```python
from build123d import *

# Parameters (mm, degrees)
SKETCH1_W           = 64.08
SKETCH1_H           = 37.749
BOSS_EXTRUDE1_DEPTH = 20.32
SKETCH1_6_W         = 59
SKETCH1_6_H         = 32.669
CUT_EXTRUDE1_DEPTH  = 17.78
SKETCH4_R           = 1.75
BOSS_EXTRUDE2_DEPTH = 8.89
SKETCH6_W           = 8
SKETCH6_H           = 3
CUT_EXTRUDE2_DEPTH  = 8.89


with BuildPart() as part:
    # Sketch1 → Boss-Extrude1 (new body)
    with BuildSketch(Plane(origin=(0, 0, 0), x_dir=(1, 0, 0), z_dir=(0, 1, 0))):
        Rectangle(SKETCH1_W, SKETCH1_H)
    extrude(amount=-BOSS_EXTRUDE1_DEPTH)

    # Sketch1_6 → Cut-Extrude1 (cut)
    with BuildSketch(Plane(origin=(0, 0, 0), x_dir=(1, 0, 0), z_dir=(0, 1, 0))):
        Rectangle(SKETCH1_6_W, SKETCH1_6_H)
    extrude(amount=-CUT_EXTRUDE1_DEPTH, mode=Mode.SUBTRACT)

    # Sketch4 → Boss-Extrude2 (add)
    # profile 1 of 4: a face of its own
    with BuildSketch(Plane(origin=(0, -17.78, 0), x_dir=(1, 0, 0), z_dir=(0, 1, 0))):
        with BuildLine():
            Line((-29.5, 16.3345), (-24.3228, 16.3345))
            ThreePointArc((-24.3228, 16.3345), (-24.192690413, 11.027190413), (-29.5, 10.897080827))
            Line((-29.5, 10.897080827), (-29.5, 16.3345))
        make_face()
        with Locations(Location((-26.9114, 13.615790413, 0), (0, 0, 270))):
            Circle(SKETCH4_R, mode=Mode.SUBTRACT)
    # profile 2 of 4: a face of its own
    with BuildSketch(Plane(origin=(0, -17.78, 0), x_dir=(1, 0, 0), z_dir=(0, 1, 0))):
        with BuildLine():
            Line((29.5, 10.897080827), (29.5, 16.3345))
            Line((29.5, 16.3345), (24.3228, 16.3345))
            ThreePointArc((24.3228, 16.3345), (24.192690413, 11.027190413), (29.5, 10.897080827))
        make_face()
        with Locations(Location((26.9114, 13.615790413, 0), (0, 0, 270))):
            Circle(SKETCH4_R, mode=Mode.SUBTRACT)
    # profile 3 of 4: a face of its own
    with BuildSketch(Plane(origin=(0, -17.78, 0), x_dir=(1, 0, 0), z_dir=(0, 1, 0))):
        with BuildLine():
            Line((29.5, -10.897080827), (29.5, -16.3345))
            Line((29.5, -16.3345), (24.3228, -16.3345))
            ThreePointArc((24.3228, -16.3345), (24.192690413, -11.027190413), (29.5, -10.897080827))
        make_face()
        with Locations(Location((26.9114, -13.615790413, 0), (0, 0, 270))):
            Circle(SKETCH4_R, mode=Mode.SUBTRACT)
    # profile 4 of 4: a face of its own
    with BuildSketch(Plane(origin=(0, -17.78, 0), x_dir=(1, 0, 0), z_dir=(0, 1, 0))):
        with BuildLine():
            Line((-29.5, -10.897080827), (-29.5, -16.3345))
            Line((-29.5, -16.3345), (-24.3228, -16.3345))
            ThreePointArc((-24.3228, -16.3345), (-24.192690413, -11.027190413), (-29.5, -10.897080827))
        make_face()
        with Locations(Location((-26.9114, -13.615790413, 0), (0, 0, 270))):
            Circle(SKETCH4_R, mode=Mode.SUBTRACT)
    extrude(amount=BOSS_EXTRUDE2_DEPTH)

    # Sketch6 → Cut-Extrude2 (cut)
    with BuildSketch(Plane(origin=(32.04, 0, 0), x_dir=(0, 0, -1), z_dir=(1, 0, 0))):
        with Locations((-0.19, -7.82)):
            Rectangle(SKETCH6_W, SKETCH6_H)
    extrude(amount=-CUT_EXTRUDE2_DEPTH, mode=Mode.SUBTRACT)


solid = part.part
```
Geometry: final body of the model. Coordinates: model frame, mm. A direction names the side the tool comes from. Coordinates: 2 decimals unless noted, no trailing zeros. Order: outer loops, then holes, each group sorted by start corner. A loop starts at its lowest first (then second) coordinate and runs counter-clockwise, first axis right, second up. Notation, with made-up numbers: M 21,-15 L 46,-15 A12 ccw 46,-9 Z; hole C -1.5,83 d1. An arc over 180 degrees is marked long. Answer as CSV lines item,"result".
Q1. Section B-B on y = -4.75. Return the cut outline in (x, z).
Answers:
outline,"M -32.04,-18.87 L 32.04,-18.87 L 32.04,18.87 L -32.04,18.87 Z; hole M -29.5,-16.33 L 29.5,-16.33 L 29.5,16.33 L -29.5,16.33 Z"
Q2. Section D-D on y = -7.5. Return the cut outline in (x, z).
Answers:
outline,"M -32.04,-18.87 L 32.04,-18.87 L 32.04,-3.81 L 29.5,-3.81 L 29.5,-16.33 L -29.5,-16.33 L -29.5,16.33 L 29.5,16.33 L 29.5,4.19 L 32.04,4.19 L 32.04,18.87 L -32.04,18.87 Z"
Q3. Draft query along Z for faces 1 (the cylindrical face through (-24.136, -13.397, 11.088)), 2 (the flat face through (-3, 0, 17)), 3 (the flat face through (0, -10, -18.874)). Return one class per face: pulls with the +Z half, pulls with the -Z half, needs draft (parallel to the pull), parting line crosses it, or undercut.
Answers:
face 1,"undercut"
face 2,"needs draft"
face 3,"pulls with the -Z half"
Q4. First-contact query: P1, Ø1, axis at x = 27, z = 13.5, coming from the +Y side; P2, Ø4, axis at x = -26.91, z = 13.62, coming from the +Y side. Flat tips, straight axial feed; report the tip coordinate or a pass-through.
Answers:
P1,"stops at y = -17.78"
P2,"stops at y = -8.89"
Q5. Section A-A on z = -2. Return the cut outline in (x, y), and give its area (3 significant figures).
Answers:
outline,"M -32.04,-20.32 L 32.04,-20.32 L 32.04,-9.32 L 29.5,-9.32 L 29.5,-17.78 L -29.5,-17.78 L -29.5,0 L -32.04,0 Z; M 29.5,-6.32 L 32.04,-6.32 L 32.04,0 L 29.5,0 Z"
area,"245 mm^2"
Q6. Line query: probe 1 along X at (y, z) = (-11.25, -8); probe 2 along Z at (x, y) = (-20, -8); probe 3 along Z at (x, y) = (-28, -14). Output: solid intervals per line, ascending. Write a range as [from, to].
Answers:
probe 1,"x = [-32.04, -29.5], [29.5, 32.04]"
probe 2,"z = [-18.87, -16.33], [16.33, 18.87]"
probe 3,"z = [-18.87, -14.99], [-12.25, -10.02], [10.02, 12.25], [14.99, 18.87]"
Q7. Section C-C on x = -15. Return the cut outline in (y, z).
Answers:
outline,"M -20.32,-18.87 L 0,-18.87 L 0,-16.33 L -17.78,-16.33 L -17.78,16.33 L 0,16.33 L 0,18.87 L -20.32,18.87 Z"
Q8. Set-up query: faces 4 (the flat face through (31, -8, -3.81)), 5 (the flat face through (29.5, -11, 0)). Return all of +Z, -Z, +X, -X, +Y, -Y with unobstructed straight access to the full face (end or side cutting, diameter ignored); none if empty.
Answers:
face 4,"+X"
face 5,"+Y"
